Geometry check sheet. Reference: the model listing, model coordinates, mm. Face numbers are marked on the shaded views. A direction names the side the tool comes from. Coordinates: 2 decimals unless noted, no trailing zeros. Order: outer loops, then holes, each group sorted by start corner. A loop starts at its lowest first (then second) coordinate and runs counter-clockwise, first axis right, second up. Notation, with made-up numbers: M -34,26.5 L 13,26.5 A33 cw 13,60.5 Z; hole C -19.75,44 d8. An arc over 180 degrees is marked long. One line per item, written item: value. Start each with the question number.
1) Thickness scan on L1, parallel to Y at x = 0, z = 5.8; L2, parallel to Z at x = -5.5, y = -2.25; L3, parallel to X at y = 8.75, z = 1.75. Record the ranges inside material, lowest first. Write a range as from..to.
2) Sectioned sample at A-A, the plane z = 4.5. Enter the section's corners in (x, y).
3) Access from +Z, -Z, +X, -X, +Y, -Y to the whole of each face (thin tool, end or side, straight path). Record for the marked faces 1 and 2.
4) Draft check along Y on the marked faces 3, 4, 5 and 6. Enter one of: pulls with the +Y half, pulls with the -Y half, needs draft (parallel to the pull), parting line crosses it, or undercut.
5) Go/stop test with flat-tipped pins: P1, Ø1.5, axis at x = 1.5, y = -7, coming from the +Z side; P2, Ø3, axis at x = 2.5, z = 1, coming from the -Y side; P3, Ø1, axis at x = -2.5, y = -4, coming from the +Z side. Record where each tip stops, or that it passes through.
```python
from build123d import *

# Parameters (mm, degrees)
F0_R      = 11
F1_DEPTH  = 3
F5_R      = 5.5
F6_DEPTH  = 1
F7_R      = 4
F8_DEPTH  = 2.9
F9_R      = 2.95
F10_DEPTH = 2.9
F11_R     = 0.3


with BuildPart() as f1:
    # F0 (on Top) → F1 (new body)
    with BuildSketch(Plane.XY):
        Circle(F0_R)
    extrude(amount=F1_DEPTH)

    # F3 (on Front) → F4 (revolve, cut)
    with BuildSketch(Plane.XZ):
        with BuildLine():
            Line((0, -42.4037037037), (0, 2.7))
            ThreePointArc((0, 2.7), (-22.5518518519, -19.8518518519), (0, -42.4037037037))
        make_face()
    revolve(axis=Axis((0, 0, -19.8518518519), (0, 0, -1)), mode=Mode.SUBTRACT)

    # F5 (on face) → F6 (join)
    with BuildSketch(Plane.XY.offset(3)):
        Circle(F5_R)
    extrude(amount=F6_DEPTH)

    # F7 (on face) → F8 (join)
    with BuildSketch(Plane.XY.offset(4)):
        Circle(F7_R)
    extrude(amount=F8_DEPTH)

    # F9 (on face) → F10 (cut)
    with BuildSketch(Plane.XY.offset(6.9)):
        Circle(F9_R)
    extrude(amount=-F10_DEPTH, mode=Mode.SUBTRACT)

    # F11
    f11_edges = [f1.edges().sort_by_distance(p)[0] for p in [
        (10.7, 0, 0),
    ]]
    fillet(f11_edges, radius=F11_R)


solid = f1.part
```
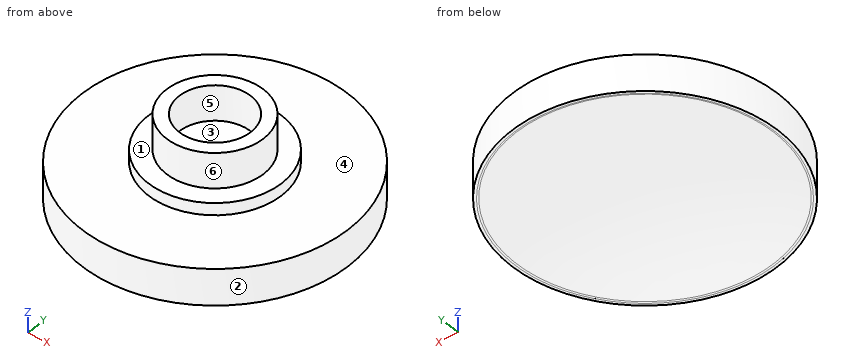
Final values:
1. L1: y = -4..-2.95, 2.95..4
1. L2: z = 1.9..3
1. L3: x = -6.67..6.67
2. outline: C 0,0 d8; hole C 0,0 d5.9
3. face 1: +Z
3. face 2: +Z, -Z
4. face 3: undercut
4. face 4: needs draft
4. face 5: undercut
4. face 6: parting line crosses it
5. P1: stops at z = 3
5. P2: stops at y = -10.95
5. P3: stops at z = 4
